from build123d import *

# Parameters (mm, degrees)
F0_W     = 116
F0_H     = 53
F1_DEPTH = 52
F3_DEPTH = 23
F4_R     = 2.5
F5_DEPTH = 8
F6_SIZE  = 5
F7_W     = 46
F7_H     = 12.914198093
F8_DEPTH = 4


# Not quite as in the source:
# - a feature names something its author has since deleted; it is built from what else it names


with BuildPart() as f1:
    # F0 (on Front) → F1 (new body)
    with BuildSketch(Plane.XZ):
        with Locations((0, 8.5)):
            Rectangle(F0_W, F0_H)
    extrude(amount=F1_DEPTH)

    # F2 (on Right) → F3 (join, symmetric)
    with BuildSketch(Plane.YZ):
        with BuildLine():
            Line((-45, 35), (0, 35))
            Line((0, 35), (0, 47.914198093))
            ThreePointArc((0, 47.914198093), (-24.3783358313, 66.3998162753), (-45, 89))
            Line((-45, 89), (-45, 35))
        make_face()
        with BuildLine():
            Line((-52, 35), (-45, 35))
            Line((-45, 35), (-45, 89))
            ThreePointArc((-45, 89), (-48.5, 89.7722433198), (-52, 89))
            Line((-52, 89), (-52, 35))
        make_face()
    extrude(amount=F3_DEPTH, both=True)

    # F4 (on face) → F5 (join)
    with BuildSketch(Plane.XZ.offset(52)):
        Polygon((-23, 89), (-79, 89), (-79, -39), (79, -39), (79, 89), (23, 89), (23, 35), (58, 35), (58, -18), (-58, -18), (-58, 35), (-23, 35), align=None)
        with Locations((0, -28.3078663051)):
            Circle(F4_R, mode=Mode.SUBTRACT)
        with Locations((-51.8612675369, 69.1157281399)):
            Circle(F4_R, mode=Mode.SUBTRACT)
        with Locations((51.8612675369, 69.1157281399)):
            Circle(F4_R, mode=Mode.SUBTRACT)
        Polygon((23, 89), (-23, 89), (-23, 35), (-58, 35), (-58, -18), (58, -18), (58, 35), (23, 35), align=None)
    extrude(amount=F5_DEPTH)

    # F6
    f6_edges = [f1.edges().sort_by_distance(p)[0] for p in [
        (-79, -56, 89),
        (79, -56, 89),
        (79, -56, -39),
        (-79, -56, -39),
    ]]
    chamfer(f6_edges, length=F6_SIZE)

    # F7 (on face) → F8 (join)
    with BuildSketch(Plane(origin=(0, 0, 0), x_dir=(-1, 0, 0), z_dir=(0, 1, 0))):
        with Locations((0, 41.4570990465)):
            Rectangle(F7_W, F7_H)
        Polygon((-23, 35), (-58, 35), (-58, -18), (58, -18), (58, 35), (23, 35), align=None)
    extrude(amount=F8_DEPTH)


solid = f1.part
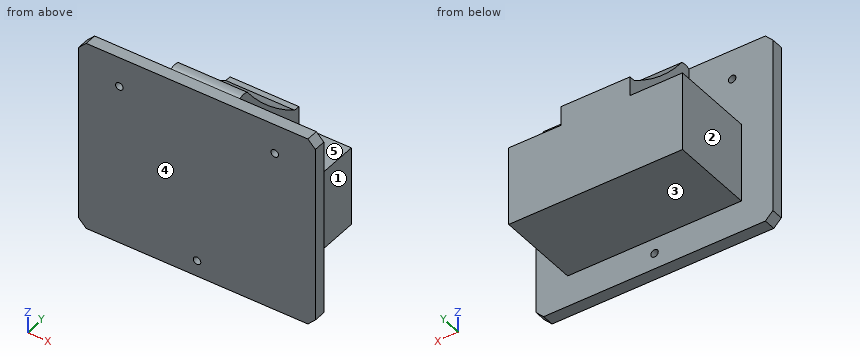
Check sheet for the modelled part. Datum: model origin and axes. Units: mm. Face numbers are marked on the shaded views. A direction names the side the tool comes from. Round coordinates to 2 decimals unless told otherwise and drop trailing zeros. Order: outer loops, then holes, each group sorted by start corner. A loop starts at its lowest first (then second) coordinate and runs counter-clockwise, first axis right, second up. Notation, with made-up numbers: M 46,89.25 L 72,89.25 A14 ccw 72,93.25 Z; hole C -7.5,16.25 d4. An arc over 180 degrees is marked long. One line per item, written item: value. Start each with the question number.
1. Section check B-B on x = 12. Enter the section's corners in (y, z).
2. Access from +Z, -Z, +X, -X, +Y, -Y to the whole of each face (thin tool, end or side, straight path). Record for the marked faces 1, 2, 3, 4 and 5.
3. Section check D-D on y = -24.5. Enter the section's corners in (x, z).
4. Section check C-C on x = -52. Enter the section's corners in (y, z), and give its area (3 significant figures).
5. Section check A-A on z = 18. Enter the section's corners in (x, y), and give its area (3 significant figures).
6. Gauge pin test, flat ends, axial feed: P1, Ø3, axis at x = 35, y = -44.5, coming from the -Z side; P2, Ø6, axis at x = -51.86, z = 69.12, coming from the +Y side; P3, Ø16.5, axis at y = -23, z = 58, coming from the +X side; P4, Ø4, axis at x = 51.86, z = 69.12, coming from the -Y side. Record the tip position at first contact, or that the pin passes through.
7. Scan lines: line 1 along Z through (x, y) = (0, -55.25); line 2 along Z through (x, y) = (55.5, -6); line 3 along Y through (x, z) = (24.5, 75). Record each from-to range of solid material in increasing order.
Results found:
1. outline: M -60,-39 L -52,-39 L -52,-18 L 4,-18 L 4,47.91 L 0,47.91 A168 cw -45,89 A8.32 ccw -52,89 L -60,89 Z
2. face 1: +Z, -Z, +X, +Y
2. face 2: +Z, -Z, -X, +Y
2. face 3: -Z, +X, -X, +Y
2. face 4: +Z, -Z, +X, -X, -Y
2. face 5: +Z, +X, +Y
3. outline: M -58,-18 L 58,-18 L 58,35 L 23,35 L 23,66.51 L -23,66.51 L -23,35 L -58,35 Z
4. outline: M -60,-39 L -52,-39 L -52,-18 L 4,-18 L 4,35 L -52,35 L -52,66.62 L -60,66.62 Z; M -60,71.61 L -52,71.61 L -52,89 L -60,89 Z
4. area: 3,950 mm^2
5. outline: M -79,-60 L 79,-60 L 79,-52 L 58,-52 L 58,4 L -58,4 L -58,-52 L -79,-52 Z
5. area: 7,760 mm^2
6. P1: z = -18
6. P2: y = -52
6. P3: x = 23
6. P4: through
7. line 1: -39 to -30.81, -25.81 to 89
7. line 2: -18 to 35
7. line 3: -60 to -52
